Part print with two shaded views. Sizes in mm from the minimum x, y, z corner. Coordinates: 2 decimals unless noted, no trailing zeros. Write each loop counter-clockwise with the first axis right and the second up, starting at its lowest first coordinate (ties: lowest second). Pieces come first, ordered by that corner, then holes.
Q1. Band-saw the part on C-C, the plane y = 5.25. Write the cut outline in (x, z).
Q2. Band-saw the part on B-B, the plane x = 19.05. Write the cut outline in (y, z).
Q3. Drill centre lines: probe 1 along X at (y, z) = (3, 70); probe 2 along Z at (x, y) = (6.35, 3); probe 3 along X at (y, z) = (5.75, 88.5). Where is each one in solid material? Low to high.
Q4. Band-saw the part on D-D, the plane x = 7.75. Write the cut outline in (y, z), plus the area to 3 significant figures.
Q5. Band-saw the part on A-A, the plane z = 10. Write the cut outline in (x, y), plus the area to 4 significant figures.
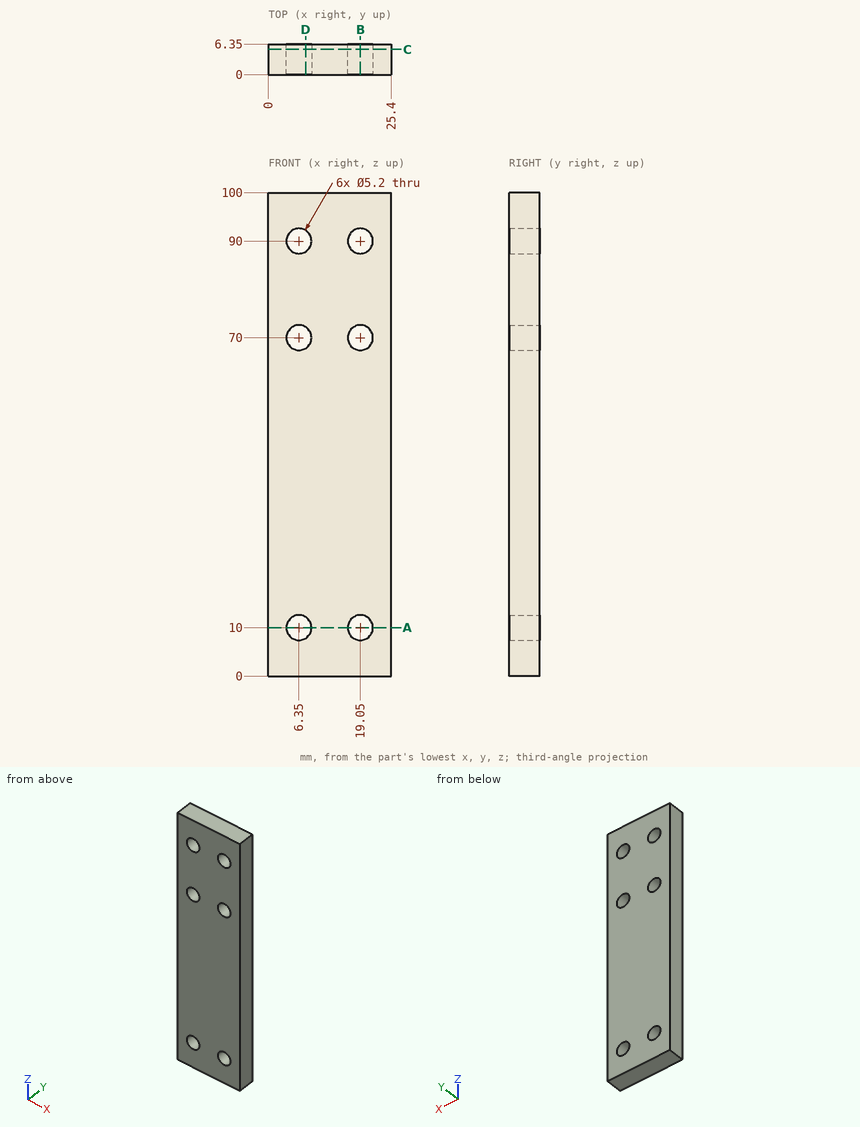
Answer sheet:
1. outline: (0, 0) - (25.4, 0) - (25.4, 100) - (0, 100) - close; hole circle Ø5.2 at (6.35, 10); hole circle Ø5.2 at (6.35, 70); hole circle Ø5.2 at (6.35, 90); hole circle Ø5.2 at (19.05, 10); hole circle Ø5.2 at (19.05, 70); hole circle Ø5.2 at (19.05, 90)
2. outline: (0, 0) - (6.35, 0) - (6.35, 7.4) - (0, 7.4) - close; (0, 12.6) - (6.35, 12.6) - (6.35, 67.4) - (0, 67.4) - close; (0, 72.6) - (6.35, 72.6) - (6.35, 87.4) - (0, 87.4) - close; (0, 92.6) - (6.35, 92.6) - (6.35, 100) - (0, 100) - close
3. probe 1: x = 0 to 3.75, 8.95 to 16.45, 21.65 to 25.4
3. probe 2: z = 0 to 7.4, 12.6 to 67.4, 72.6 to 87.4, 92.6 to 100
3. probe 3: x = 0 to 4.23, 8.47 to 16.93, 21.17 to 25.4
4. outline: (0, 0) - (6.35, 0) - (6.35, 7.81) - (0, 7.81) - close; (0, 12.19) - (6.35, 12.19) - (6.35, 67.81) - (0, 67.81) - close; (0, 72.19) - (6.35, 72.19) - (6.35, 87.81) - (0, 87.81) - close; (0, 92.19) - (6.35, 92.19) - (6.35, 100) - (0, 100) - close
4. area: 552 mm2
5. outline: (0, 0) - (3.75, 0) - (3.75, 6.35) - (0, 6.35) - close; (8.95, 0) - (16.45, 0) - (16.45, 6.35) - (8.95, 6.35) - close; (21.65, 0) - (25.4, 0) - (25.4, 6.35) - (21.65, 6.35) - close
5. area: 95.25 mm2
